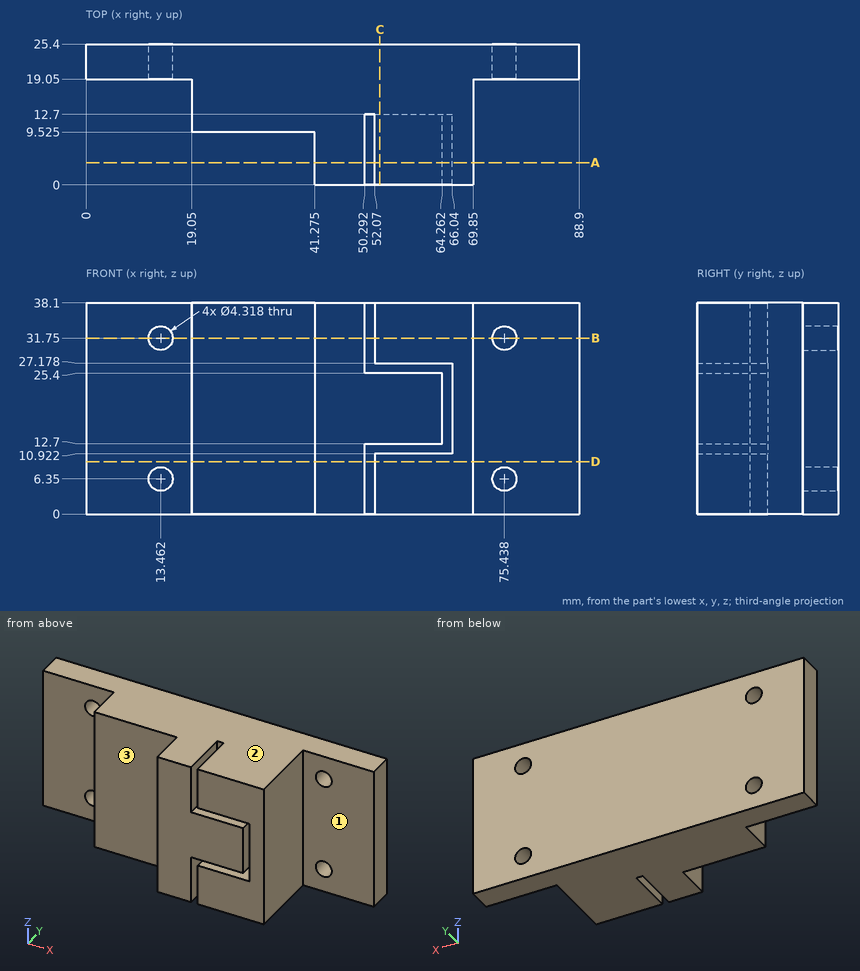
Study the drawing (mm; zero at the part's minimum x, y, z) and answer. A direction names the side the tool comes from. Give positions to 0.01 mm unless a question says otherwise; leave off trailing zeros. Write each loop counter-clockwise with the first axis right and the second up, starting at its lowest first coordinate (ties: lowest second). Pieces come first, ordered by that corner, then holes. Notation, with made-up numbers: (-25.75, 51.5) -> (23.25, 51.5) arc R31 cw to (23.25, 76.5) -> close; hole circle Ø9 at (54.5, -12.75). An arc over 180 degrees is marked (long way). Answer as a JSON object with one key per item and string values. Group by question number.
1) Find section A-A (y = 4). Write down the section's boundary in (x, z) (3 decimals), and give its area (3 significant figures).
2) Find section C-C (x = 53). Write down the section's boundary in (y, z), and give its area (3 significant figures).
3) Each of these flat-tipped pins is pushed along its axis until it touches: P1, Ø4, axis at x = 13.462, z = 6.35, coming from the +Y side (1 decimal); P2, Ø21, axis at x = 75, z = 19, coming from the -Y side; P3, Ø6.5, axis at y = 4, z = 34, coming from the +X side; P4, Ø6, axis at x = 77.5, z = 25.5, coming from the -Y side. Where does it stop, or does it pass through?
4) Find section B-B (z = 31.75). Write down the section's boundary in (x, y) (3 decimals), and give its area (3 significant figures).
5) Find section D-D (z = 9.5). Write down the section's boundary in (x, y) (3 decimals), and give its area (3 significant figures).
6) A tool of negligible diameter and unlimited length cuts with its end or side. For the marked faces 1, 2 and 3, from which of +Z, -Z, +X, -X, +Y, -Y can it reach the whole face along a straight path? Write none if from no direction.
7) Consider L1, parallel to X at y = 22.5, z = 31.75; L2, parallel to Z at x = 60, y = 3.5; L3, parallel to X at y = 5.5, z = 13 (3 decimals). Determine where each line is inside the solid, lowest interval first. Write a range as from..to.
Values follow:
{
 "1": {"outline": "(41.275, 0) -> (50.292, 0) -> (50.292, 12.7) -> (64.262, 12.7) -> (64.262, 25.4) -> (50.292, 25.4) -> (50.292, 38.1) -> (41.275, 38.1) -> close; (52.07, 0) -> (69.85, 0) -> (69.85, 38.1) -> (52.07, 38.1) -> (52.07, 27.178) -> (66.04, 27.178) -> (66.04, 10.922) -> (52.07, 10.922) -> close", "area": "971 mm2"},
 "2": {"outline": "(0, 0) -> (25.4, 0) -> (25.4, 38.1) -> (0, 38.1) -> (0, 27.18) -> (12.7, 27.18) -> (12.7, 25.4) -> (0, 25.4) -> (0, 12.7) -> (12.7, 12.7) -> (12.7, 10.92) -> (0, 10.92) -> close", "area": "923 mm2"},
 "3": {"P1": "passes through", "P2": "stops at y = 0", "P3": "stops at x = 69.85", "P4": "stops at y = 19.05"},
 "4": {"outline": "(0, 19.05) -> (11.303, 19.05) -> (11.303, 25.4) -> (0, 25.4) -> close; (15.621, 19.05) -> (19.05, 19.05) -> (19.05, 9.525) -> (41.275, 9.525) -> (41.275, 0) -> (50.292, 0) -> (50.292, 12.7) -> (52.07, 12.7) -> (52.07, 0) -> (69.85, 0) -> (69.85, 19.05) -> (73.279, 19.05) -> (73.279, 25.4) -> (15.621, 25.4) -> close; (77.597, 19.05) -> (88.9, 19.05) -> (88.9, 25.4) -> (77.597, 25.4) -> close", "area": "1,240 mm2"},
 "5": {"outline": "(0, 19.05) -> (19.05, 19.05) -> (19.05, 9.525) -> (41.275, 9.525) -> (41.275, 0) -> (50.292, 0) -> (50.292, 12.7) -> (52.07, 12.7) -> (52.07, 0) -> (69.85, 0) -> (69.85, 19.05) -> (88.9, 19.05) -> (88.9, 25.4) -> (0, 25.4) -> close", "area": "1,300 mm2"},
 "6": {"face 1": "+Z, -Z, +X, -Y", "face 2": "+Z, +X, -X, +Y, -Y", "face 3": "+Z, -Z, -X, -Y"},
 "7": {"L1": "x = 0..11.3, 15.62..73.28, 77.6..88.9", "L2": "z = 0..10.92, 12.7..25.4, 27.18..38.1", "L3": "x = 41.275..64.262, 66.04..69.85"}
}
